Design review of the part built by this model. Coordinates are the model's own, in mm. Face numbers are marked on the shaded views. A direction names the side the tool comes from. Coordinates: 2 decimals unless noted, no trailing zeros. Loops run counter-clockwise (first coordinate to the right, second up) from the corner with the lowest first, then second, coordinate; pieces in that order, holes last. Notation, with made-up numbers: (51, 46.25) -> (64, 46.25) arc R22 ccw to (64, 85.25) -> close; hole circle Ø9 at (60, 45.5). An arc over 180 degrees is marked (long way). Answer in a Markdown table with one row per item.
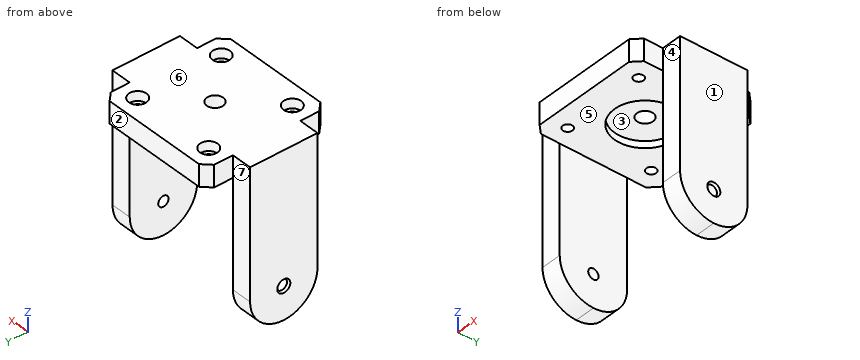
Solid Edge part; units mm, degrees
sketch "Sketch1" plane through (0, 0, 0) normal (0, 0, 1) x (1, 0, 0)
  line L0 (-22.5, -22.5) -> (22.5, -22.5)
  line L1 (22.5, -22.5) -> (22.5, 22.5)
  line L2 (22.5, 22.5) -> (-22.5, 22.5)
  line L3 (-22.5, 22.5) -> (-22.5, -22.5)
  dimension "D1" = 22.5
extrude "Protrusion1" add sketch "Sketch1" along normal mid plane 8
hole "Hole_1" at (-15.5, 15.5, 4) direction (0, 0, -1) diameter 3.6 end up to next counterbore diameter 6.5 counterbore depth 3.5
hole "Hole1" at (15.5, 15.5, 4) direction (0, 0, -1) diameter 3.6 end up to next counterbore diameter 6.5 counterbore depth 3.5
hole "Hole2" at (-15.5, -15.5, 4) direction (0, 0, -1) diameter 3.6 end up to next counterbore diameter 6.5 counterbore depth 3.5
hole "Hole3" at (15.5, -15.5, 4) direction (0, 0, -1) diameter 3.6 end up to next counterbore diameter 6.5 counterbore depth 3.5
chamfer "Chamfer_1" distance 3 angle 45 4 edges at (-22.5, -22.5, 0) (-22.5, 22.5, 0) (22.5, 22.5, 0) (22.5, -22.5, 0)
hole "Hole_5" at (0, 0, -4) direction (0, 0, 1) diameter 6 end up to next counterbore diameter 22.5 counterbore depth 2.5
sketch "Sketch2" plane through (22.5, 0, 0) normal (1, 0, 0) x (0, -1, 0)
  line L0 (-12.5, -4) -> (12.5, -4)
  line L1 (12.5, -4) -> (12.5, 56)
  line L2 (12.5, 56) -> (-12.5, 56)
  line L3 (-12.5, 56) -> (-12.5, -4)
  dimension "D1" = 12.5
  dimension "D2" = 12.5
extrude "ExtrudedProtrusion_2" add sketch "Sketch2" along normal blind 7.5
hole "Hole_6" at (30, 0, -44) direction (-1, 0, 0) diameter 3.85 end up to next
fillet "Round_1" radius 12.5 2 edges at (26.25, -12.5, -56) (26.25, 12.5, -56)
mirror "Mirror1" about plane through (0, 0, 0) normal (1, 0, 0) of "ExtrudedProtrusion_2", "Hole_6"
fillet "Round1" radius 12.5 2 edges at (-26.25, -12.5, -56) (-26.25, 12.5, -56)
chamfer "Chamfer_2" distance 0.5 angle 60 2 edges at (-30, 1.925, -44) (30, 1.925, -44) measured on face at (30, 8.0833, -46.6) measured on face at (-30, 8.0833, -46.6)
properties material "Polyethylene, low density"
(1) Draft analysis for pull direction Y (two halves, no side actions). For the marked faces 1, 2 and 3, state which applies: pulls with the +Y half, pulls with the -Y half, needs draft (parallel to the pull), parting line crosses it, or undercut.
Evaluation:
| item | result |
|---|---|
| face 1 | needs draft |
| face 2 | pulls with the +Y half |
| face 3 | undercut |
(2) To check wall thickness, follow probe 1 along X at (y, z) = (15.5, -1.7); probe 2 along X at (y, z) = (15.5, 2.6). State the ranges of each line that lie inside material, in increasing order.
Evaluation:
| item | result |
|---|---|
| probe 1 | x = -22.5 to -17.3, -13.7 to 13.7, 17.3 to 22.5 |
| probe 2 | x = -22.5 to -18.75, -12.25 to 12.25, 18.75 to 22.5 |
(3) For pin 1 (2 mm diameter, centred on x = -26, z = -21.5, fed in from +Y); pin 2 (2 mm diameter, centred on y = 16.5, z = -1.5, fed in from +X); pin 3 (4 mm diameter, centred on x = 23, z = -49.5, fed in from +Y), all flat-tipped, find the tip position at first contact; note any pin that passes through.
Evaluation:
| item | result |
|---|---|
| pin 1 | stops at y = 12.5 |
| pin 2 | stops at x = 22.5 |
| pin 3 | stops at y = 11.84 |
(4) Take a section at B-B on z = -25.5. Give the boundary of the cut face in (x, y), and give its area (3 significant figures).
Evaluation:
| item | result |
|---|---|
| outline | (-30, -12.5) -> (-22.5, -12.5) -> (-22.5, 12.5) -> (-30, 12.5) -> close; (22.5, -12.5) -> (30, -12.5) -> (30, 12.5) -> (22.5, 12.5) -> close |
| area | 375 mm² |
(5) Tool access review of the marked faces 4, 5, 6 and 7: name each direction out of +Z, -Z, +X, -X, +Y, -Y from which nothing blocks a thin tool from reaching the whole face with its end or side.
Evaluation:
| item | result |
|---|---|
| face 4 | +Z, -Z, +X, -Y |
| face 5 | -Z, +Y, -Y |
| face 6 | +Z, +X, -X, +Y, -Y |
| face 7 | +Z, -Z, -X, +Y |
(6) Take a section at A-A on x = 0. Give the boundary of the cut face in (y, z), and give its area (3 significant figures).
Evaluation:
| item | result |
|---|---|
| outline | (-22.5, -4) -> (-11.25, -4) -> (-11.25, -1.5) -> (-3, -1.5) -> (-3, 4) -> (-22.5, 4) -> close; (3, -1.5) -> (11.25, -1.5) -> (11.25, -4) -> (22.5, -4) -> (22.5, 4) -> (3, 4) -> close |
| area | 271 mm² |
(7) Take a section at C-C on x = -15.5. Give the boundary of the cut face in (y, z).
Evaluation:
| item | result |
|---|---|
| outline | (-22.5, -4) -> (-17.3, -4) -> (-17.3, 0.5) -> (-18.75, 0.5) -> (-18.75, 4) -> (-22.5, 4) -> close; (-13.7, -4) -> (13.7, -4) -> (13.7, 0.5) -> (12.25, 0.5) -> (12.25, 4) -> (-12.25, 4) -> (-12.25, 0.5) -> (-13.7, 0.5) -> close; (17.3, -4) -> (22.5, -4) -> (22.5, 4) -> (18.75, 4) -> (18.75, 0.5) -> (17.3, 0.5) -> close |
